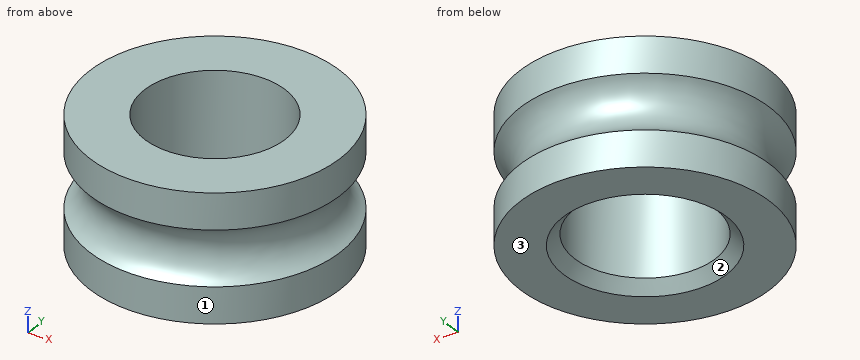
```python
from build123d import *

# Parameters (mm, degrees)
F2_SIZE = 0.8


with BuildPart() as f1:
    # F0 (on Front) → F1 (revolve)
    with BuildSketch(Plane.XZ):
        with BuildLine():
            Line((5, 9), (5, 0))
            Line((5, 0), (8.875, 0))
            Line((8.875, 0), (8.875, 2.551443))
            ThreePointArc((8.875, 2.551443), (7.75, 4.5), (8.875, 6.448557))
            Line((8.875, 6.448557), (8.875, 9))
            Line((8.875, 9), (5, 9))
        make_face()
    revolve(axis=Axis((0, 0, 23.187623), (0, 0, 1)))

    # F2
    f2_edges = [f1.edges().sort_by_distance(p)[0] for p in [
        (-5, 0, 0),
    ]]
    chamfer(f2_edges, length=F2_SIZE)


solid = f1.part
```
Design review of the part built by this model. Coordinates are the model's own, in mm. Face numbers are marked on the shaded views. Round coordinates to 2 decimals unless told otherwise and drop trailing zeros. Order: outer loops, then holes, each group sorted by start corner. A loop starts at its lowest first (then second) coordinate and runs counter-clockwise, first axis right, second up. Notation, with made-up numbers: M 8.5,-37.75 L 15.5,-37.75 A33 ccw 15.5,-4.75 Z; hole C -13.75,-6 d2. An arc over 180 degrees is marked long. Put each result on its own line as item: value.
Q1. To check wall thickness, follow line 1 (Y direction, x = 0, z = 7) (3 decimals); line 2 (Y direction, x = 0, z = 3.5); line 3 (Z direction, x = -4.25, y = -7.25). State the ranges of each line that lie inside material, in increasing order.
Reported:
line 1: -8.875 to -5, 5 to 8.875
line 2: -7.98 to -5, 5 to 7.98
line 3: 0 to 2.91, 6.09 to 9
Q2. Draft analysis for pull direction Y (two halves, no side actions). For the marked faces 1, 2 and 3, state which applies: released by +Y, released by -Y, zero draft, split by the parting line, or undercut.
Reported:
face 1: split by the parting line
face 2: undercut
face 3: zero draft
Q3. Consider section A-A (x = 0). State the section outline as (y, z) points (3 decimals).
Reported:
outline: M -8.875,0 L -5.8,0 L -5,0.8 L -5,9 L -8.875,9 L -8.875,6.449 A2.25 cw -8.875,2.551 Z; M 5,0.8 L 5.8,0 L 8.875,0 L 8.875,2.551 A2.25 cw 8.875,6.449 L 8.875,9 L 5,9 Z
Q4. Insertion check: pin 1 Ø1.5 at (x, z) = (-4.5, 4) entering from -Y; pin 2 Ø8 at (x, y) = (0, 0) entering from -Z (3 decimals); pin 3 Ø4 at (y, z) = (5.5, 6) entering from +X; pin 4 Ø4 at (y, z) = (-4.5, 6) entering from +X. Each pin has a flat end and moves straight along its axis. Give the tip position at first contact, or say it passes through.
Reported:
pin 1: y = -6.95
pin 2: through
pin 3: x = 8.13
pin 4: x = 8.5
Q5. Consider section D-D (z = 3.25). State the section outline as (x, y) points.
Reported:
outline: C 0,0 d16.26; hole C 0,0 d10
Q6. Consider section C-C (z = 2.25). State the section outline as (x, y) points (3 decimals), and give its area (3 significant figures).
Reported:
outline: C 0,0 d17.75; hole C 0,0 d10
area: 169 mm²
